```python
from build123d import *

# Parameters (mm, degrees)
F1_DEPTH = 152.4
F3_DEPTH = 76.2


with BuildPart() as f1:
    # F0 (on Right) → F1 (new body)
    with BuildSketch(Plane.YZ):
        Polygon((25.4, 50.8), (0, 50.8), (0, 0), (76.2, 0), (76.2, 50.8), (50.8, 50.8), (50.8, 38.1), (63.5, 38.1), (63.5, 25.4), (12.7, 25.4), (12.7, 38.1), (25.4, 38.1), align=None)
    extrude(amount=F1_DEPTH)

    # F2 (on face) → F3 (cut, through all)
    with BuildSketch(Plane.XZ):
        Polygon((114.3, 0), (127, 12.7), (25.48896, 12.7), (38.1, 0), align=None)
    extrude(amount=-F3_DEPTH, mode=Mode.SUBTRACT)


solid = f1.part
```
Check sheet for the modelled part. Datum: model origin and axes. Units: mm. A direction names the side the tool comes from. Coordinates: 2 decimals unless noted, no trailing zeros. Write each loop counter-clockwise with the first axis right and the second up, starting at its lowest first coordinate (ties: lowest second). Pieces come first, ordered by that corner, then holes. Notation, with made-up numbers: (43, 77.5) -> (58, 77.5) arc R16 ccw to (58, 83.5) -> close; hole circle Ø6 at (33.5, 47). An arc over 180 degrees is marked (long way). Use a Markdown table: item, result.
1. Release check for a two-part mould opening along Z. For faces 6 (the flat face through (133, 38, 0)), 7 (the flat face through (75, 50.8, 45)), 8 (the flat face through (75, 63.5, 32)) record: pulls with the +Z half, pulls with the -Z half, needs draft (parallel to the pull), parting line crosses it, or undercut.
Reported:
| item | result |
|---|---|
| face 6 | pulls with the -Z half |
| face 7 | needs draft |
| face 8 | undercut |
2. Scan lines: line 1 along Y through (x, z) = (121.5, 37.5); line 2 along Y through (x, z) = (57, 46); line 3 along Z through (x, y) = (115, 61.5). Record each from-to range of solid material in increasing order.
Reported:
| item | result |
|---|---|
| line 1 | y = 0 to 12.7, 63.5 to 76.2 |
| line 2 | y = 0 to 25.4, 50.8 to 76.2 |
| line 3 | z = 0 to 0.7, 12.7 to 25.4, 38.1 to 50.8 |
3. Sectioned sample at D-D (x = 29.5). Enter the section's corners in (y, z).
Reported:
| item | result |
|---|---|
| outline | (0, 0) -> (76.2, 0) -> (76.2, 8.66) -> (0, 8.66) -> close; (0, 12.7) -> (76.2, 12.7) -> (76.2, 50.8) -> (50.8, 50.8) -> (50.8, 38.1) -> (63.5, 38.1) -> (63.5, 25.4) -> (12.7, 25.4) -> (12.7, 38.1) -> (25.4, 38.1) -> (25.4, 50.8) -> (0, 50.8) -> close |
4. Tool access check on faces 1 (the flat face through (31.706, 37.567, 6.439)), 2 (the flat face through (75, 25.4, 44)), 3 (the flat face through (75, 13, 50.8)), 4 (the flat face through (75, 12.7, 32)), 5 (the flat face through (19, 38, 0)). Record the directions out of +Z, -Z, +X, -X, +Y, -Y that give a thin tool (end or side, any length) a straight path to the whole face; none if there is none.
Reported:
| item | result |
|---|---|
| face 1 | +Y, -Y |
| face 2 | +Z, +X, -X |
| face 3 | +Z, +X, -X, +Y, -Y |
| face 4 | +X, -X |
| face 5 | -Z, +X, -X, +Y, -Y |
5. Sectioned sample at B-B (x = 72). Enter the section's corners in (y, z).
Reported:
| item | result |
|---|---|
| outline | (0, 12.7) -> (76.2, 12.7) -> (76.2, 50.8) -> (50.8, 50.8) -> (50.8, 38.1) -> (63.5, 38.1) -> (63.5, 25.4) -> (12.7, 25.4) -> (12.7, 38.1) -> (25.4, 38.1) -> (25.4, 50.8) -> (0, 50.8) -> close |
6. Sectioned sample at A-A (z = 44.5). Enter the section's corners in (x, y), plus the area to 3 significant figures.
Reported:
| item | result |
|---|---|
| outline | (0, 0) -> (152.4, 0) -> (152.4, 25.4) -> (0, 25.4) -> close; (0, 50.8) -> (152.4, 50.8) -> (152.4, 76.2) -> (0, 76.2) -> close |
| area | 7,740 mm2 |
7. Sectioned sample at C-C (y = 7). Enter the section's corners in (x, z), plus the area to 3 significant figures.
Reported:
| item | result |
|---|---|
| outline | (0, 0) -> (38.1, 0) -> (25.49, 12.7) -> (127, 12.7) -> (114.3, 0) -> (152.4, 0) -> (152.4, 50.8) -> (0, 50.8) -> close |
| area | 6,610 mm2 |
8. Go/stop test with a flat-tipped pin: pin 1 Ø10 at (x, y) = (73.5, 21) entering from -Z. Record where the tip stops, or that it passes through.
Reported:
| item | result |
|---|---|
| pin 1 | stops at z = 12.7 |
